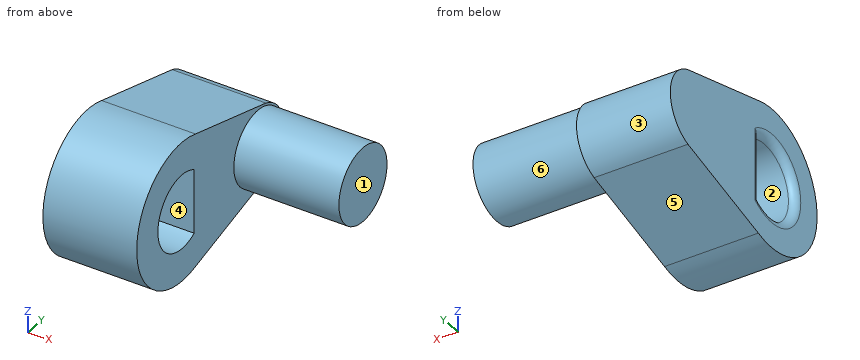
```python
from build123d import *

# Parameters (mm, degrees)
BOSS_EXTRUDE2_DEPTH = 2.5
SKETCH4_R           = 0.99
CUT_EXTRUDE2_DEPTH  = 64.988660757
SKETCH6_R           = 0.99
BOSS_EXTRUDE4_DEPTH = 2.8
SKETCH7_W           = 2.01987101
SKETCH7_H           = 0.78494751
BOSS_EXTRUDE5_DEPTH = 2.5
FILLET1_R           = 0.2


with BuildPart() as part:
    # Sketch3 → Boss-Extrude2 (new body)
    with BuildSketch(Plane(origin=(0, 0, 0), x_dir=(0, 0, -1), z_dir=(1, 0, 0))):
        with BuildLine():
            Line((-54.67077374, 30.968825597), (-55.447230875, 28.071048118))
            ThreePointArc((-55.447230875, 28.071048118), (-53.67077374, 25.652507451), (-51.894316605, 28.071048118))
            Line((-51.894316605, 28.071048118), (-52.67077374, 30.968825597))
            ThreePointArc((-52.67077374, 30.968825597), (-53.67077374, 31.692969852), (-54.67077374, 30.968825597))
        make_face()
    extrude(amount=BOSS_EXTRUDE2_DEPTH)

    # Sketch4 → Cut-Extrude2 (cut, through all)
    with BuildSketch(Plane(origin=(2.5, 0, 0), x_dir=(0, 0, -1), z_dir=(1, 0, 0))):
        with Locations((-53.67077374, 27.514195996)):
            Circle(SKETCH4_R)
    extrude(amount=-CUT_EXTRUDE2_DEPTH, mode=Mode.SUBTRACT)

    # Sketch6 → Boss-Extrude4 (add)
    with BuildSketch(Plane(origin=(2.5, 0, 0), x_dir=(0, 0, -1), z_dir=(1, 0, 0))):
        with Locations((-53.67077374, 30.640427563)):
            Circle(SKETCH6_R)
    extrude(amount=BOSS_EXTRUDE4_DEPTH)

    # Sketch7 → Boss-Extrude5 (add)
    with BuildSketch(Plane(origin=(2.5, 0, 0), x_dir=(0, 0, -1), z_dir=(1, 0, 0))):
        with Locations((-53.657499813, 28.408869671)):
            Rectangle(SKETCH7_W, SKETCH7_H)
    extrude(amount=-BOSS_EXTRUDE5_DEPTH)

    # Fillet1
    fillet1_edges = [part.edges().sort_by_distance(p)[0] for p in [
        (0, 26.524195996, 53.67077374),
        (0, 28.016395916, 53.67077374),
    ]]
    fillet(fillet1_edges, radius=FILLET1_R)


solid = part.part
```
Source: CAD feature listing. Evaluate the final solid. Frame: model axes, mm. Face numbers are marked on the shaded views. A direction names the side the tool comes from. Coordinates: 2 decimals unless noted, no trailing zeros. Order: outer loops, then holes, each group sorted by start corner. A loop starts at its lowest first (then second) coordinate and runs counter-clockwise, first axis right, second up. Notation, with made-up numbers: M 35.25,23 L 84.25,23 A27 cw 84.25,59 Z; hole C 89,6 d9. An arc over 180 degrees is marked long. Write each question's results on one line, items separated by ' | '. Start each with the question number.
1) Section query A-A (x = 2.2). Return the cut outline in (y, z), plus the area to 3 significant figures.
2) Section query C-C (z = 52.25). Return the cut outline in (x, y).
3) Line query: line 1 (Z direction, x = 0.85, y = 26.75); line 2 (X direction, y = 28.25, z = 53.05); line 3 (Y direction, x = 4.05, z = 53.7). Output: solid intervals per line, ascending. Write a range as from..to.
4) Section query D-D (y = 28.5). Return the cut outline in (x, z), plus the area to 3 significant figures.
5) Access query for the marked faces 4, 5 and 6. Directions: +Z, -Z, +X, -X, +Y, -Y. A direction counts if a zero-diameter tool reaches every point of the face in a straight line with its end or side. Return the directions, or none.
6) Draft query along Y for the marked faces 1, 2 and 3. Return one class per face: released by +Y, released by -Y, zero draft, split by the parting line, or undercut.
7) Contact query for a flat-ended pin moving along its axis: pin 1 Ø1.9 at (y, z) = (28, 54.5) entering from +X. Output: stop coordinate, or through.
8) Section query B-B (y = 30.5). Return the cut outline in (x, z).
Answers:
1) outline: M 28.07,51.89 L 30.97,52.67 A1.05 ccw 30.97,54.67 L 28.07,55.45 A1.86 ccw long Z; hole M 28.02,52.82 L 28.02,54.52 A0.99 ccw long Z | area: 14.1 mm^2
2) outline: M 0,26.31 L 2.5,26.31 L 2.5,29.4 L 0,29.4 Z
3) line 1: z = 51.97..53.04, 54.3..55.37 | line 2: x = 0..2.5 | line 3: y = 29.65..31.63
4) outline: M 0,52.01 L 2.5,52.01 L 2.5,55.33 L 0,55.33 Z | area: 8.31 mm^2
5) face 4: +X, -X | face 5: -Z, +X, -X, +Y | face 6: +X
6) face 1: zero draft | face 2: undercut | face 3: released by +Y
7) pin 1: stops at x = 2.5
8) outline: M 0,52.55 L 2.5,52.55 L 2.5,52.69 L 5.3,52.69 L 5.3,54.65 L 2.5,54.65 L 2.5,54.8 L 0,54.8 Z
